The model under review builds one solid part; all positions refer to its coordinate system, in mm. Face numbers are marked on the shaded views. A direction names the side the tool comes from. Round coordinates to 2 decimals unless told otherwise and drop trailing zeros. Write each loop counter-clockwise with the first axis right and the second up, starting at its lowest first coordinate (ties: lowest second). Pieces come first, ordered by that corner, then holes. Notation, with made-up numbers: (-21.5, -20) -> (7.5, -20) arc R15 ccw to (7.5, -14) -> close; hole circle Ø9 at (-9.75, 26). An arc over 180 degrees is marked (long way). Return JSON: item names as keys, results as strings. Group by question number.
1. For line 1 along Y through (x, z) = (0, 41.75) (3 decimals); line 2 along Y through (x, z) = (0, 37) (3 decimals); line 3 along Z through (x, y) = (1.25, 5.5), list the stretches that pass through material, from the lowest coordinate up. Write a range as from..to.
2. Clearance check with flat-ended pins moving along their axes: P1, Ø6.5, axis at x = -1.5, z = 28.5, coming from the -Y side; P2, Ø1, axis at x = -5, z = 40, coming from the +Y side; P3, Ø6, axis at y = 4.5, z = 16.5, coming from the +X side. State where each tip first meets the part, or that it passes through.
3. Take a section at C-C, the plane y = 4.25. Write out the cut boundary in (x, z).
4. Mouldability with a two-part tool opening along Y and no side actions: class the marked faces 1, 2 and 3 as pulls with the +Y half, pulls with the -Y half, needs draft (parallel to the pull), parting line crosses it, or undercut.
5. Tool access review of the marked faces 4 and 5: name each direction out of +Z, -Z, +X, -X, +Y, -Y from which nothing blocks a thin tool from reaching the whole face with its end or side.
6. Take a section at B-B, the plane x = 5. Write out the cut boundary in (y, z).
7. Take a section at A-A, the plane z = 4.5. Write out the cut boundary in (x, y), then the cut area to 3 significant figures.
Autodesk Inventor part; units mm, degrees
ref_plane "Work Plane1" through (-6.35, 0, 0) normal (1, 0, 0) x (0, 1, 0)
ref_plane "XZ Plane" through (0, 0, 0) normal (0, 1, 0) x (-1, 0, 0)
ref_plane "XY Plane" through (0, 0, 0) normal (0, 0, 1) x (1, 0, 0)
sketch "Sketch1" plane through (0, 0, 0) normal (0, 0, 1) x (1, 0, 0)
  circle A0 centre (0, 0) radius 6.35
  dimension "d0" = 12.7
extrude "Extrusion1" add sketch "Sketch1" along normal blind 52.07
ref_plane "Work Plane1" through (-6.35, 0, 0) normal (1, 0, 0) x (0, 1, 0)
sketch "Sketch2" plane through (-6.35, 0, 0) normal (1, 0, 0) x (0, 1, 0)
  line L0 (-6.35, 0) -> (6.35, 0)
  line L1 (6.35, 52.07) -> (-6.35, 52.07)
  line L2 (6.35, 0) -> (6.35, 52.07)
  line L3 (-6.35, 0) -> (-6.35, 52.07)
  line L4 (6.35, 20.32) -> (5, 20.32)
  line L5 (5, 20.32) -> (5, 39.37)
  line L6 (5, 39.37) -> (6.35, 39.37)
  line L7 (6.35, 39.37) -> (6.35, 20.32)
  line L8 (-6.35, 20.32) -> (-5, 20.32)
  line L9 (-5, 20.32) -> (-5, 39.37)
  line L10 (-5, 39.37) -> (-6.35, 39.37)
  line L11 (-6.35, 39.37) -> (-6.35, 20.32)
  point P0 (0, 0)
  dimension "d3" = 19.05
  dimension "d4" = 12.7
  dimension "d5" = 10
extrude "Extrusion2" cut sketch "Sketch2" along normal mid plane 52.07 contours L3 L10 L9 L8 | L4 L5 L6 L2
sketch "Sketch3" plane through (0, 0, 52.07) normal (0, 0, 1) x (1, 0, 0)
  point P0 (0, 0)
  point P1 (0, 0)
hole "Hole1" at (0, 0, 52.07) direction (0, 0, -1) diameter 6.35 depth 25.4 tip angle 118
properties part number "Pin V2"
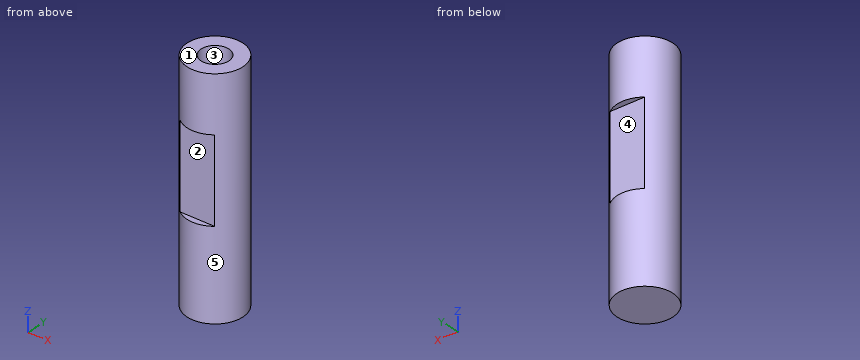
Output:
{
 "1": {"line 1": "y = -6.35..-3.175, 3.175..6.35", "line 2": "y = -5..-3.175, 3.175..5", "line 3": "z = 0..20.32, 39.37..52.07"},
 "2": {"P1": "stops at y = -5", "P2": "stops at y = 4.48", "P3": "stops at x = 6.17"},
 "3": {"outline": "(-4.72, 0) -> (4.72, 0) -> (4.72, 52.07) -> (-4.72, 52.07) -> close"},
 "4": {"face 1": "needs draft", "face 2": "pulls with the -Y half", "face 3": "undercut"},
 "5": {"face 4": "+X, -X, +Y", "face 5": "+Z, -Z"},
 "6": {"outline": "(-3.91, 0) -> (3.91, 0) -> (3.91, 52.07) -> (-3.91, 52.07) -> close"},
 "7": {"outline": "circle Ø12.7 at (0, 0)", "area": "127 mm^2"}
}
